from build123d import *

# Parameters (mm, degrees)
SKETCH_1_R          = 4.575
SKETCH_1_W          = 6.9
SKETCH_1_H          = 10.08
SKETCH_1_R_2        = 1.2
EXTRUDE_1_DEPTH     = 2
EXTRUDE_2_DEPTH     = 4.125036756
SKETCH_3_W          = 1.88
SKETCH_3_H          = 14.24
CUT_EXTRUDE_1_DEPTH = 4.125036756
SKETCH_4_W          = 6.9
SKETCH_4_H          = 0.56
SKETCH_4_H_2        = 0.55
EXTRUDE_3_DEPTH     = 4.125036756
SKETCH_5_W          = 0.215
SKETCH_5_H          = 23.05
CUT_EXTRUDE_2_DEPTH = 4.125036756
SKETCH_6_W          = 0.745
SKETCH_6_H          = 2.575
SKETCH_6_W_2        = 6.9
EXTRUDE_4_DEPTH     = 2
SKETCH_7_R          = 5.5
SKETCH_7_R_2        = 4.575
EXTRUDE_5_DEPTH     = 12
CHAMFER_1_SIZE      = 0.6
SKETCH_8_R          = 6.5
SKETCH_8_R_2        = 5.5
EXTRUDE_6_DEPTH     = 2
EXTRUDE_7_DEPTH     = 15.935
SKETCH_10_W         = 36.02
SKETCH_10_H         = 4.455
EXTRUDE_8_DEPTH     = 3.53
CHAMFER_3_SIZE      = 2
CHAMFER_4_SIZE      = 2
CUT_EXTRUDE_4_DEPTH = 10


with BuildPart() as part:
    # 草图1 → 凸台-拉伸1 (new body)
    # profile 1 of 2: a face of its own
    with BuildSketch(Plane.XY):
        Polygon((83.862310964, 7.15), (85.802310964, 7.15), (85.802310964, 13.83), (83.862310964, 13.83), (83.862310964, 25.12), (77.212310964, 25.12), (77.212310964, 30), (66.372310964, 30), (66.372310964, 25.12), (59.662310964, 25.12), (59.662310964, 25.076338502), (59.782310964, 25), (59.782310964, -34.93), (83.862310964, -34.93), align=None)
        with Locations((71.792310964, -25.065)):
            Circle(SKETCH_1_R, mode=Mode.SUBTRACT)
        with Locations((71.792310964, -0.89)):
            Rectangle(SKETCH_1_W, SKETCH_1_H, mode=Mode.SUBTRACT)
        with Locations((71.792310964, 13.19)):
            Rectangle(SKETCH_1_W, SKETCH_1_H, mode=Mode.SUBTRACT)
    # profile 2 of 2: a face of its own
    with BuildSketch(Plane.XY):
        Polygon((85.802310964, -27.361541817), (85.802310964, 7.15), (83.862310964, 7.15), (83.862310964, -34.93), (59.782310964, -34.93), (59.782310964, 25), (59.662310964, 25.076338502), (59.662310964, 25.12), (66.372310964, 25.12), (66.372310964, 30), (77.212310964, 30), (77.212310964, 25.12), (83.862310964, 25.12), (83.862310964, 13.83), (85.802310964, 13.83), (85.802310964, 21.12), (89.802310964, 25.12), (89.802310964, 29.961541817), (88.402310964, 31.361541817), (49.782310964, 31.361541817), (49.782310964, -31.361541817), (57.782310964, -36.93), (88.402310964, -36.93), (89.802310964, -35.53), (89.802310964, -31.361541817), align=None)
        with Locations((52.782310964, -28.361541817)):
            Circle(SKETCH_1_R_2, mode=Mode.SUBTRACT)
        with Locations((87.802310964, -34.145770908)):
            Circle(SKETCH_1_R_2, mode=Mode.SUBTRACT)
        with Locations((52.782310964, 28.361541817)):
            Circle(SKETCH_1_R_2, mode=Mode.SUBTRACT)
        with Locations((87.802310964, 28.240770908)):
            Circle(SKETCH_1_R_2, mode=Mode.SUBTRACT)
    extrude(amount=EXTRUDE_1_DEPTH)

    # 草图2 → 凸台-拉伸2 (add)
    with BuildSketch(Plane.XY.offset(2)):
        Polygon((79.187310964, 17.68), (79.187310964, 19.56), (65.717310964, 19.56), (65.717310964, 15.155), (59.717310964, 15.155), (59.717310964, -2.845), (65.717310964, -2.845), (65.717310964, -7.25), (79.187310964, -7.25), (79.187310964, -5.37), (75.242310964, -5.37), (75.242310964, -5.93), (68.342310964, -5.93), (68.342310964, -5.37), (67.597310964, -5.37), (67.597310964, -0.965), (61.597310964, -0.965), (61.597310964, 13.275), (67.597310964, 13.275), (67.597310964, 17.68), (68.342310964, 17.68), (68.342310964, 18.23), (75.242310964, 18.23), (75.242310964, 17.68), align=None)
        Polygon((83.187310964, 17.68), (83.187310964, 19.56), (79.187310964, 19.56), (79.187310964, 17.68), (81.067310964, 17.68), (81.307310964, 17.68), align=None)
        Polygon((85.802310964, 19.56), (83.187310964, 19.56), (83.187310964, 17.68), (85.587310964, 17.68), (85.587310964, -5.37), (83.187310964, -5.37), (83.187310964, -7.25), (85.802310964, -7.25), align=None)
        Polygon((79.187310964, -7.25), (83.187310964, -7.25), (83.187310964, -5.37), (81.307310964, -5.37), (81.067310964, -5.37), (79.187310964, -5.37), align=None)
    extrude(amount=EXTRUDE_2_DEPTH)

    # 草图3 → 切除-拉伸1 (cut)
    with BuildSketch(Plane.XY.offset(6.125036756)):
        with Locations((60.657310964, 6.155)):
            Rectangle(SKETCH_3_W, SKETCH_3_H)
    extrude(amount=-CUT_EXTRUDE_1_DEPTH, mode=Mode.SUBTRACT)

    # 草图4 → 凸台-拉伸3 (add)
    with BuildSketch(Plane.XY.offset(6.125036756)):
        with Locations((71.792310964, -5.65)):
            Rectangle(SKETCH_4_W, SKETCH_4_H)
        with Locations((71.792310964, 17.955)):
            Rectangle(SKETCH_4_W, SKETCH_4_H_2)
    extrude(amount=-EXTRUDE_3_DEPTH)

    # 草图5 → 切除-拉伸2 (cut)
    with BuildSketch(Plane.XY.offset(6.125036756)):
        with Locations((85.694810964, 6.155)):
            Rectangle(SKETCH_5_W, SKETCH_5_H)
    extrude(amount=-CUT_EXTRUDE_2_DEPTH, mode=Mode.SUBTRACT)

    # 草图6 → 凸台-拉伸4 (add)
    with BuildSketch(Plane.XY.offset(6.125036756)):
        Polygon((67.597310964, -5.37), (67.597310964, -2.795), (65.717310964, -2.795), (65.717310964, -2.845), (65.717310964, -7.25), (67.597310964, -7.25), align=None)
        Polygon((85.802310964, -5.37), (75.242310964, -5.37), (68.342310964, -5.37), (67.597310964, -5.37), (67.597310964, -7.25), (85.802310964, -7.25), align=None)
        with Locations((67.969810964, -4.0825)):
            Rectangle(SKETCH_6_W, SKETCH_6_H)
        with Locations((71.792310964, -4.0825)):
            Rectangle(SKETCH_6_W_2, SKETCH_6_H)
        Polygon((85.467310964, -2.795), (81.187310964, -2.795), (75.242310964, -2.795), (75.242310964, -5.37), (85.802310964, -5.37), (85.802310964, -2.795), align=None)
        Polygon((65.717310964, 15.105), (67.597310964, 15.105), (67.597310964, 17.68), (67.597310964, 19.56), (65.717310964, 19.56), (65.717310964, 15.155), align=None)
        Polygon((68.342310964, 17.68), (75.242310964, 17.68), (85.802310964, 17.68), (85.802310964, 19.56), (67.597310964, 19.56), (67.597310964, 17.68), align=None)
        with Locations((67.969810964, 16.3925)):
            Rectangle(SKETCH_6_W, SKETCH_6_H)
        with Locations((71.792310964, 16.3925)):
            Rectangle(SKETCH_6_W_2, SKETCH_6_H)
        Polygon((75.242310964, 15.105), (81.187310964, 15.105), (85.467310964, 15.105), (85.802310964, 15.105), (85.802310964, 17.68), (75.242310964, 17.68), align=None)
    extrude(amount=EXTRUDE_4_DEPTH)

    # 草图7 → 凸台-拉伸5 (add)
    with BuildSketch(Plane.XY.offset(2)):
        with Locations((71.792310964, -25.065)):
            Circle(SKETCH_7_R)
        with Locations((71.792310964, -25.065)):
            Circle(SKETCH_7_R_2, mode=Mode.SUBTRACT)
    extrude(amount=EXTRUDE_5_DEPTH)

    # 倒角1
    chamfer_1_edges = [part.edges().sort_by_distance(p)[0] for p in [
        (67.217310964, -25.065, 0),
    ]]
    chamfer(chamfer_1_edges, length=CHAMFER_1_SIZE)

    # 草图8 → 凸台-拉伸6 (add)
    with BuildSketch(Plane.XY.offset(2)):
        with Locations((71.792310964, -25.065)):
            Circle(SKETCH_8_R)
        with Locations((71.792310964, -25.065)):
            Circle(SKETCH_8_R_2, mode=Mode.SUBTRACT)
    extrude(amount=EXTRUDE_6_DEPTH)

    # 草图9 → 凸台-拉伸7 (add)
    with BuildSketch(Plane.ZY.offset(-65.717310964)):
        Polygon((2, -7.25), (8.125036756, -7.25), (8.125036756, -2.795), (6.125036756, -2.795), (6.125036756, -2.845), (2, -2.845), align=None)
        Polygon((2, 15.155), (6.125036756, 15.155), (6.125036756, 15.105), (8.125036756, 15.105), (8.125036756, 19.56), (2, 19.56), align=None)
    extrude(amount=EXTRUDE_7_DEPTH)

    # 草图10 → 凸台-拉伸8 (add)
    with BuildSketch(Plane.XY.offset(8.125036756)):
        with Locations((67.792310964, -5.0225)):
            Rectangle(SKETCH_10_W, SKETCH_10_H)
        with Locations((67.792310964, 17.3325)):
            Rectangle(SKETCH_10_W, SKETCH_10_H)
    extrude(amount=EXTRUDE_8_DEPTH)

    # 倒角3
    chamfer_3_edges = [part.edges().sort_by_distance(p)[0] for p in [
        (67.792310964, 19.56, 11.655036756),
        (67.792310964, -7.25, 11.655036756),
        (67.792310964, 19.56, 2),
        (67.792310964, -7.25, 2),
    ]]
    chamfer(chamfer_3_edges, length=CHAMFER_3_SIZE)

    # 倒角4
    chamfer_4_edges = [part.edges().sort_by_distance(p)[0] for p in [
        (65.292310964, -25.065, 2),
    ]]
    chamfer(chamfer_4_edges, length=CHAMFER_4_SIZE - 0.0001)  # a hair under: the kernel refuses the full size

    # 草图12 → 切除-拉伸4 (cut)
    with BuildSketch(Plane.XY.offset(2)):
        Polygon((75.242310964, 8.15), (75.242310964, 4.15), (75.242310964, -5.37), (85.802310964, -5.37), (85.802310964, 17.68), (75.242310964, 17.68), align=None)
    extrude(amount=-CUT_EXTRUDE_4_DEPTH, mode=Mode.SUBTRACT)


solid = part.part
Verification items for the finished model (mm, model axes). A direction names the side the tool comes from. Give positions to 0.01 mm unless a question says otherwise; leave off trailing zeros. Order: outer loops, then holes, each group sorted by start corner. A loop starts at its lowest first (then second) coordinate and runs counter-clockwise, first axis right, second up. Notation, with made-up numbers: M -34,55 L -29,55 A15 cw -29,64 Z; hole C 9.25,33.5 d3. An arc over 180 degrees is marked long. Answer as a JSON object with one key per item and string values. Group by question number.
1) Cross-section at C-C (x = 69). Give the number of separate pieces and of enclosed holes in the cut face, then the cut area to 3 significant figures.
2) Cross-section at A-A (z = 3.25). Enter the section's corners in (x, y) (3 decimals).
3) Cross-section at D-D (z = 12.75). Enter the section's corners in (x, y) (3 decimals), then the cut area to 3 significant figures.
4) Scan lines: line 1 along Y through (x, z) = (57, 9.25) (3 decimals); line 2 along Y through (x, z) = (80, 6); line 3 along X through (y, z) = (7, 1.5). Record each from-to range of solid material in increasing order. Write a range as [from, to].
5) Mould release check, pull along Y, two halves, no side actions. Record for faces 1 (the face through (65, -2, 0)), 2 (the face through (69, 31.362, 1)), 3 (the face through (64, -0.965, 4)): released by +Y, released by -Y, zero draft, split by the parting line, or undercut.
6) Access from +Z, -Z, +X, -X, +Y, -Y to the whole of each face (thin tool, end or side, straight path). Record for faces 4 (the face through (68, 19.56, 7)), 5 (the face through (72, 8.15, 1)), 6 (the face through (67.54, -6.236, 10.669)), 7 (the face through (72, 18.23, 1)).
7) Depth check by flat-ended pin: pin 1 Ø5 at (x, y) = (57, -11) entering from -Z; pin 2 Ø2 at (x, z) = (59, 11) entering from +Y; pin 3 Ø0.8 at (x, y) = (74.5, -4.5) entering from -Z; pin 4 Ø0.5 at (x, y) = (63, 14) entering from +Z. Enter the tip coordinate at first touch or a pass-through.
8) Cross-section at B-B (y = 26). Enter the section's corners in (x, z).
Result sheet:
{
 "1": {"separate pieces": "4", "enclosed holes": "0", "area": "182 mm2"},
 "2": {"outline": "M 49.782,-8 L 85.802,-8 L 85.802,-5.37 L 67.597,-5.37 L 67.597,-0.965 L 59.717,-0.965 L 59.717,-2.845 L 49.782,-2.845 Z; M 49.782,15.155 L 59.717,15.155 L 59.717,13.275 L 67.597,13.275 L 67.597,17.68 L 85.802,17.68 L 85.802,20.31 L 49.782,20.31 Z; C 71.792,-25.065 d14.5; hole C 71.792,-25.065 d9.15"},
 "3": {"outline": "C 71.792,-25.065 d11; hole C 71.792,-25.065 d9.15", "area": "29.3 mm2"},
 "4": {"line 1": "y = [-7.25, -2.795], [15.105, 19.56]", "line 2": "y = [-7.25, -5.37], [17.68, 19.56]", "line 3": "x = [49.78, 75.24]"},
 "5": {"face 1": "zero draft", "face 2": "released by +Y", "face 3": "undercut"},
 "6": {"face 4": "+Z, +X, -X, +Y", "face 5": "+Z, -Z, +X", "face 6": "+Z, +X, -X", "face 7": "-Z"},
 "7": {"pin 1": "stops at z = 0", "pin 2": "stops at y = 19.22", "pin 3": "stops at z = 6.13", "pin 4": "stops at z = 6.13"},
 "8": {"outline": "M 49.78,0 L 89.8,0 L 89.8,2 L 49.78,2 Z"}
}
